Check sheet for the drawn part. Datum: minimum x, y, z corner. Units: mm. A direction names the side the tool comes from. Coordinates: 2 decimals unless noted, no trailing zeros. Order: outer loops, then holes, each group sorted by start corner. A loop starts at its lowest first (then second) coordinate and runs counter-clockwise, first axis right, second up. Notation, with made-up numbers: (77, 43) - (91, 43) arc R10 cw to (91, 54) - close; hole circle Ø2 at (68, 68.5). An arc over 180 degrees is marked (long way). Return JSON: item names as keys, results as strings. Group by question number.
Item 1: Gauge pin test, flat end, axial feed: pin 1 (8 mm diameter, centred on y = 39, z = 32, fed in from -X). Record the tip position at first contact, or that the pin passes through.
Item 2: Section check C-C on x = 221. Enter the section's corners in (y, z), then the cut area to 3 significant figures.
Item 3: Section check A-A on x = 279.4. Give the number of separate pieces and of enclosed holes in the cut face, then the cut area to 3 significant figures.
Item 4: Scan lines: probe 1 along Z at (x, y) = (190.5, 1.05); probe 2 along Z at (x, y) = (164, 30); probe 3 along X at (y, z) = (2, 19.05). Record each from-to range of solid material in increasing order.
Item 5: Section check B-B on x = 190.5. Enter the section's corners in (y, z).
Item 6: Tool access check on the marked faces 1 and 2. Record the directions out of +Z, -Z, +X, -X, +Y, -Y that give a thin tool (end or side, any length) a straight path to the whole face; none if there is none.
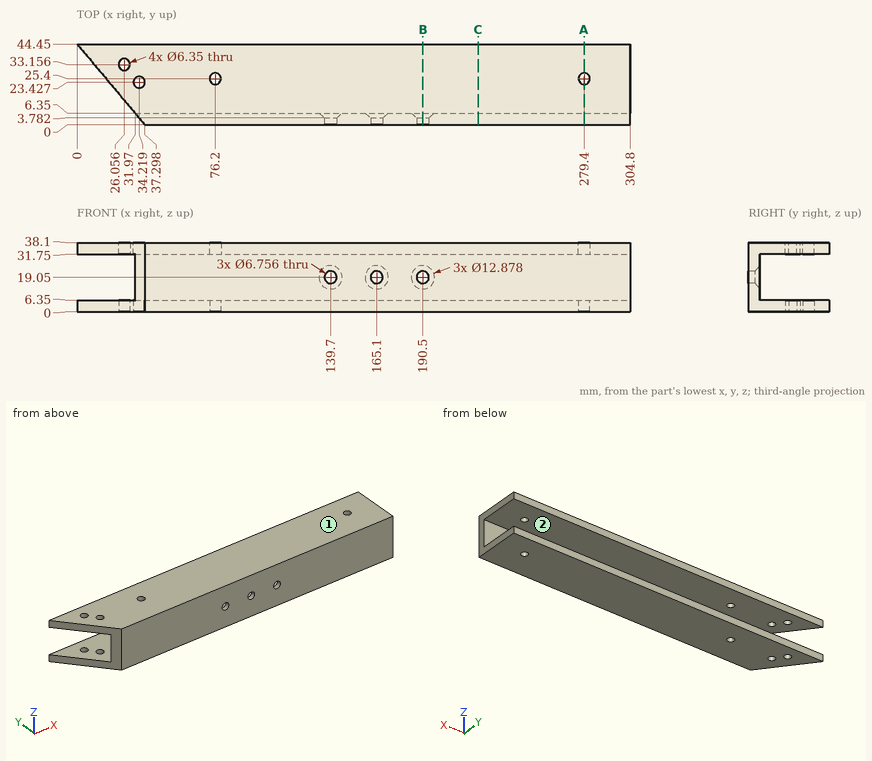
Computed:
{
 "1": {"pin 1": "stops at x = 1.22"},
 "2": {"outline": "(0, 0) - (44.45, 0) - (44.45, 6.35) - (6.35, 6.35) - (6.35, 31.75) - (44.45, 31.75) - (44.45, 38.1) - (0, 38.1) - close", "area": "726 mm²"},
 "3": {"separate pieces": "3", "enclosed holes": "0", "area": "645 mm²"},
 "4": {"probe 1": "z = 0 to 15.67, 22.43 to 38.1", "probe 2": "z = 0 to 6.35, 31.75 to 38.1", "probe 3": "x = 35.62 to 136.32, 143.08 to 161.72, 168.48 to 187.12, 193.88 to 304.8"},
 "5": {"outline": "(0, 0) - (44.45, 0) - (44.45, 6.35) - (6.35, 6.35) - (6.35, 12.61) - (3.78, 15.67) - (0, 15.67) - close; (0, 22.43) - (3.78, 22.43) - (6.35, 25.49) - (6.35, 31.75) - (44.45, 31.75) - (44.45, 38.1) - (0, 38.1) - close"},
 "6": {"face 1": "+Z, +X, -X, +Y, -Y", "face 2": "+X, -X, +Y"}
}
